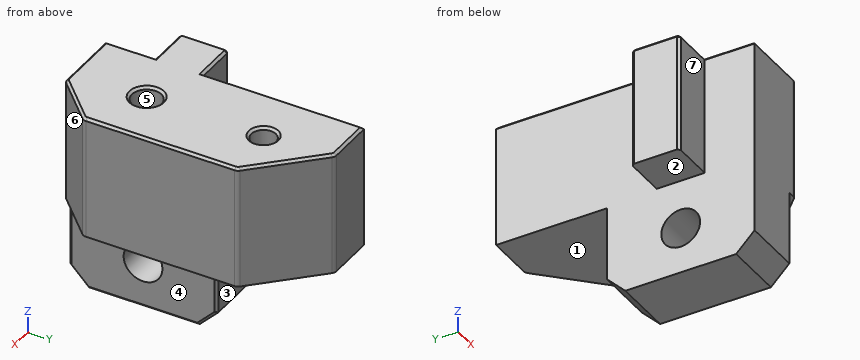
```python
from build123d import *

# Parameters (mm, degrees)
BOX016_W          = 10
BOX016_H          = 10
BOX016_DEPTH      = 17
CYLINDER004_R     = 2.4
CYLINDER004_DEPTH = 35
CYLINDER003_R     = 2
CYLINDER003_DEPTH = 30
CYLINDER008_R     = 3.15
CYLINDER008_DEPTH = 14
BOX007_W          = 7
BOX007_H          = 7.8
BOX007_DEPTH      = 20
CHAMFER005_SIZE   = 0.4
BOX006_W          = 10
BOX006_H          = 24
BOX006_DEPTH      = 15
CHAMFER004_SIZE   = 3
CHAMFER011_SIZE   = 0.4
BOX_W             = 1
BOX_H             = 7.8
BOX_DEPTH         = 15
BOX008_W          = 18
BOX008_H          = 42
BOX008_DEPTH      = 20
CHAMFER_SIZE      = 7
CHAMFER010_SIZE   = 10
FILLET002_R       = 1
CHAMFER013_SIZE   = 0.4


with BuildPart() as cube016:
    # Box016 → Box016 (new body)
    with BuildSketch(Plane(origin=(-10, 10, -16.5), x_dir=(1, 0, 0), z_dir=(0, 0, 1))):
        with Locations((5, 5)):
            Rectangle(BOX016_W, BOX016_H)
    extrude(amount=BOX016_DEPTH)


with BuildPart() as cylinder004:
    # Cylinder004 → Cylinder004 (new body)
    with BuildSketch(Plane(origin=(9, 15, 5), x_dir=(1, 0, 0), z_dir=(0, 0, 1))):
        Circle(CYLINDER004_R)
    extrude(amount=CYLINDER004_DEPTH)


with BuildPart() as cylinder003:
    # Cylinder003 → Cylinder003 (new body)
    with BuildSketch(Plane(origin=(9, 34, 10), x_dir=(1, 0, 0), z_dir=(0, 0, 1))):
        Circle(CYLINDER003_R)
    extrude(amount=CYLINDER003_DEPTH)


with BuildPart() as cylinder008:
    # Cylinder008 → Cylinder008 (new body)
    with BuildSketch(Plane(origin=(-2, 15, -7.5), x_dir=(0, 0, -1), z_dir=(1, 0, 0))):
        Circle(CYLINDER008_R)
    extrude(amount=CYLINDER008_DEPTH)


with BuildPart() as chamfer005:
    # Box007 → Box007 (new body)
    with BuildSketch(Plane(origin=(-7, 11.1, 0), x_dir=(1, 0, 0), z_dir=(0, 0, 1))):
        with Locations((3.5, 3.9)):
            Rectangle(BOX007_W, BOX007_H)
    extrude(amount=BOX007_DEPTH)

    # Chamfer005
    chamfer005_edges = [chamfer005.edges().sort_by_distance(p)[0] for p in [
        (-7, 11.1, 10),
        (-7, 18.9, 10),
    ]]
    chamfer(chamfer005_edges, length=CHAMFER005_SIZE)


with BuildPart() as chamfer011:
    # Box006 → Box006 (new body)
    with BuildSketch(Plane(origin=(0, 3, -15), x_dir=(1, 0, 0), z_dir=(0, 0, 1))):
        with Locations((5, 12)):
            Rectangle(BOX006_W, BOX006_H)
    extrude(amount=BOX006_DEPTH)

    # Chamfer004
    chamfer004_edges = [chamfer011.edges().sort_by_distance(p)[0] for p in [
        (5, 3, -15),
        (5, 27, -15),
    ]]
    chamfer(chamfer004_edges, length=CHAMFER004_SIZE)

    # Chamfer011
    chamfer011_edges = [chamfer011.edges().sort_by_distance(p)[0] for p in [
        (10, 3, -6),
        (10, 4.5, -13.5),
        (10, 15, -15),
        (10, 27, -6),
        (10, 25.5, -13.5),
    ]]
    chamfer(chamfer011_edges, length=CHAMFER011_SIZE)


with BuildPart() as cube:
    # Box → Box (new body)
    with BuildSketch(Plane(origin=(-1, 11.1, -15), x_dir=(1, 0, 0), z_dir=(0, 0, 1))):
        with Locations((0.5, 3.9)):
            Rectangle(BOX_W, BOX_H)
    extrude(amount=BOX_DEPTH)


with BuildPart() as cut002002002007004004001005:
    # Box008 → Box008 (new body)
    with BuildSketch(Plane(origin=(0, 3, 0), x_dir=(1, 0, 0), z_dir=(0, 0, 1))):
        with Locations((9, 21)):
            Rectangle(BOX008_W, BOX008_H)
    extrude(amount=BOX008_DEPTH)

    # Chamfer
    chamfer_edges = [cut002002002007004004001005.edges().sort_by_distance(p)[0] for p in [
        (18, 3, 10),
    ]]
    chamfer(chamfer_edges, length=CHAMFER_SIZE)

    # Chamfer010
    chamfer010_edges = [cut002002002007004004001005.edges().sort_by_distance(p)[0] for p in [
        (18, 45, 10),
    ]]
    chamfer(chamfer010_edges, length=CHAMFER010_SIZE)

    # Fillet002
    fillet002_edges = [cut002002002007004004001005.edges().sort_by_distance(p)[0] for p in [
        (18, 35, 10),
        (18, 10, 10),
        (8, 45, 10),
        (11, 3, 10),
    ]]
    fillet(fillet002_edges, radius=FILLET002_R)

    # Fusion: union Chamfer005, Chamfer011, Cube
    add(chamfer005.part)
    add(chamfer011.part)
    add(cube.part)

    # Cut: cut Cylinder008
    add(cylinder008.part, mode=Mode.SUBTRACT)

    # Cut002002002008: cut Cylinder003
    add(cylinder003.part, mode=Mode.SUBTRACT)

    # Cut002002002009: cut Cylinder004
    add(cylinder004.part, mode=Mode.SUBTRACT)

    # Chamfer013
    chamfer013_edges = [cut002002002007004004001005.edges().sort_by_distance(p)[0] for p in [
        (-7, 15, 20),
        (-6.8, 18.7, 20),
        (-6.8, 11.3, 20),
        (3.792893, 45, 20),
        (17.92388, 10.03153, 20),
        (14.5, 6.5, 20),
        (10.96847, 3.07612, 20),
        (7.96847, 44.92388, 20),
        (13, 40, 20),
        (17.92388, 34.96847, 20),
        (18, 22.5, 20),
        (-3.3, 11.1, 20),
        (-3.3, 18.9, 20),
        (0, 7.05, 20),
        (0, 31.95, 20),
        (5.292893, 3, 20),
        (6.6, 15, 20),
        (7, 34, 20),
    ]]
    chamfer(chamfer013_edges, length=CHAMFER013_SIZE)

    # Cut002002002007004004001005: cut Cube016
    add(cube016.part, mode=Mode.SUBTRACT)


solid = cut002002002007004004001005.part
```
Geometry check sheet. Reference: the model listing, model coordinates, mm. Face numbers are marked on the shaded views. A direction names the side the tool comes from. Round coordinates to 2 decimals unless told otherwise and drop trailing zeros. Write each loop counter-clockwise with the first axis right and the second up, starting at its lowest first coordinate (ties: lowest second). Pieces come first, ordered by that corner, then holes. Notation, with made-up numbers: (40.25, 24) -> (89.25, 24) arc R8 cw to (89.25, 31) -> close; hole circle Ø1 at (19, -19.5). An arc over 180 degrees is marked (long way). Put each result on its own line as item: value.
1) Cross-section at D-D, the plane x = 4. Enter the section's corners in (y, z).
Recorded:
outline: (3, -12) -> (6, -15) -> (24, -15) -> (27, -12) -> (27, 0) -> (45, 0) -> (45, 19.6) -> (44.6, 20) -> (3.4, 20) -> (3, 19.6) -> close; hole circle Ø6.3 at (15, -7.5)
2) Depth check by flat-ended pin: P1, Ø8, axis at y = 15, z = -7.5, coming from the +X side; P2, Ø3, axis at x = 14, y = 31.5, coming from the -Z side; P3, Ø1.2, axis at x = 8.5, y = 33.5, coming from the +Z side. Enter the tip coordinate at first touch or a pass-through.
Recorded:
P1: stops at x = 10
P2: stops at z = 0
P3: stops at z = 10
3) Access from +Z, -Z, +X, -X, +Y, -Y to the whole of each face (thin tool, end or side, straight path). Record for the marked faces 1, 2, 3 and 4.
Recorded:
face 1: -Z, +X, +Y
face 2: -Z, -X, +Y, -Y
face 3: -Z, +X, -X, +Y
face 4: -Z, +X, +Y, -Y
4) Cross-section at A-A, the plane z = -7.5. Enter the section's corners in (x, y).
Recorded:
outline: (0, 3) -> (9.6, 3) -> (10, 3.4) -> (10, 11.85) -> (0, 11.85) -> close; (0, 18.15) -> (10, 18.15) -> (10, 26.6) -> (9.6, 27) -> (0, 27) -> close
5) Release check for a two-part mould opening along X. For the marked faces 5, 6 and 7 record: pulls with the +X half, pulls with the -X half, needs draft (parallel to the pull), parting line crosses it, or undercut.
Recorded:
face 5: undercut
face 6: pulls with the +X half
face 7: needs draft
6) Thickness scan on probe 1 along X at (y, z) = (15, 13); probe 2 along Y at (x, z) = (9, 17.5); probe 3 along Y at (x, z) = (2.5, -7.5). Record the ranges inside material, lowest first. Write a range as from..to.
Recorded:
probe 1: x = -7..6.6, 11.4..18
probe 2: y = 3..12.6, 17.4..32, 36..44
probe 3: y = 3..11.85, 18.15..27
7) Cross-section at B-B, the plane z = 6. Enter the section's corners in (x, y), plus the area to 3 significant figures.
Recorded:
outline: (-7, 11.5) -> (-6.6, 11.1) -> (0, 11.1) -> (0, 3) -> (10.59, 3) arc R1 ccw to (11.29, 3.29) -> (17.71, 9.71) arc R1 ccw to (18, 10.41) -> (18, 34.59) arc R1 ccw to (17.71, 35.29) -> (8.29, 44.71) arc R1 ccw to (7.59, 45) -> (0, 45) -> (0, 18.9) -> (-6.6, 18.9) -> (-7, 18.5) -> close; hole circle Ø4.8 at (9, 15)
area: 718 mm2
8) Cross-section at C-C, the plane y = 15. Enter the section's corners in (x, z).
Recorded:
outline: (-7, 0.5) -> (0, 0.5) -> (0, -4.35) -> (10, -4.35) -> (10, 0) -> (18, 0) -> (18, 19.6) -> (17.6, 20) -> (11.8, 20) -> (11.4, 19.6) -> (11.4, 5) -> (6.6, 5) -> (6.6, 19.6) -> (6.2, 20) -> (-6.6, 20) -> (-7, 19.6) -> close; (0, -15) -> (9.6, -15) -> (10, -14.6) -> (10, -10.65) -> (0, -10.65) -> close
